Part model, mm, in its own coordinate system. A direction names the side the tool comes from. Coordinates: 2 decimals unless noted, no trailing zeros. Loops run counter-clockwise (first coordinate to the right, second up) from the corner with the lowest first, then second, coordinate; pieces in that order, holes last. Notation, with made-up numbers: (28, 10) - (45, 10) arc R26 cw to (45, 43) - close; hole circle Ø2 at (66.25, 46). An arc over 180 degrees is marked (long way). Use a Markdown table: item, result. Add a question column.
1) Band-saw the part on A-A (x = 5). Give the cut face in (y, z).
2) Probe probe 1 along Y at (x, z) = (0, -36.5); probe 2 along Z at (x, y) = (-2, 8); probe 3 along X at (y, z) = (-3.5, -16). List the from-to ranges inside material, lowest first. Write a range as [from, to].
3) Drop flat-ended pins along their axis: P1, Ø4.5, axis at x = 9.5, y = 0, coming from the +Z side; P2, Ø6.5, axis at x = 0, y = 10.5, coming from the +Z side; P3, Ø12, axis at x = 0.5, y = -0.5, coming from the -Z side; P4, Ø6, axis at x = -16, y = 10, coming from the +Z side. Give the stop position or say it passes through.
4) Pull direction Z, two halves, no side cores. Call faces 1 (the face through (-32, -7, -1)), 2 (the face through (10, 1, -13)), 3 (the face through (6.1, 10, -22)): +Z half, -Z half, draft (parallel to the pull), parting line (faces both ways), or undercut.
5) Band-saw the part on C-C (y = 4.25). Give the cut face in (x, z), plus the area to 3 significant figures.
6) Band-saw the part on D-D (z = -4). Give the cut face in (x, y).
7) Tool access for faces 4 (the face through (-13, -6.5, -3)), 5 (the face through (-13, 0, -13.3)), 6 (the face through (7, 0, -17.5)): list every direction of +Z, -Z, +X, -X, +Y, -Y with a clear straight run to the whole face (end or side of a thin tool).
8) Band-saw the part on B-B (z = -31). Give the cut face in (x, y), plus the area to 3 significant figures.
Autodesk Inventor part; units mm, degrees
ref_plane "作業平面2" through (0, 0, -13.3) normal (0, 0, 1) x (1, 0, 0)
ref_plane "作業平面3" through (0, 0, -9) normal (0, 0, 1) x (1, 0, 0)
ref_plane "作業平面4" through (-12.5, -8.5, -11.1) normal (-1, 0, 0) x (0, 0, 1)
sketch "スケッチ1" plane through (0, 0, 0) normal (0, 0, 1) x (1, 0, 0)
  circle A0 centre (0, 0) radius 1.5
  circle A1 centre (0, 0) radius 4
  line L0 (6.1, 4) -> (6.1, -4)
  line L1 (-27.76, 0) -> (17.46, 0) construction
  line L2 (6.1, 4) -> (0, 4)
  line L3 (6.1, -4) -> (0, -4)
  line L4 (6.1, -4) -> (8.1, -4)
  line L5 (8.1, -4) -> (8.1, 4)
  line L6 (8.1, 4) -> (6.1, 4)
  line L7 (0, -13.6) -> (0, 18.6) construction
  circle A2 centre (0, 10) radius 1.5
  circle A3 centre (0, 10) radius 4
  line L8 (6.1, 14) -> (6.1, 6)
  line L9 (6.1, 14) -> (0, 14)
  line L10 (6.1, 6) -> (0, 6)
  line L11 (6.1, 6) -> (8.1, 6)
  line L12 (8.1, 6) -> (8.1, 14)
  line L13 (8.1, 14) -> (6.1, 14)
  line L14 (-16.4, 6.05) -> (6.1, 6.05) construction
  line L15 (6.1, 6.05) -> (6.1, -6.05)
  line L16 (6.1, -6.05) -> (-16.4, -6.05) construction
  line L17 (-16.4, -6.05) -> (-16.4, 6.05)
  line L18 (-16.4, 6.05) -> (6.1, -6.05) construction
  line L19 (6.1, 6.05) -> (-16.4, -6.05) construction
  line L20 (-21.3, 6.05) -> (11, 6.05) construction
  line L21 (11, 6.05) -> (11, -6.05) construction
  line L22 (11, -6.05) -> (-21.3, -6.05)
  line L23 (-21.3, -6.05) -> (-21.3, 6.05) construction
  line L24 (-21.3, 6.05) -> (11, -6.05) construction
  line L25 (11, 6.05) -> (-21.3, -6.05) construction
  line L26 (-21.3, 0) -> (11, 0) construction
  circle A4 centre (-19, 0) radius 1.1
  line L27 (-5.15, 6.05) -> (-5.15, -6.05) construction
  circle A5 centre (0, 0) radius 2.425
  circle A6 centre (0, 0) radius 6.05
  circle A7 centre (0, 0) radius 9
  line L28 (8.1, -7) -> (-21.3, -7)
  line L29 (-21.3, -7) -> (-21.3, 6.05)
  line L30 (-21.3, 6.05) -> (8.1, 6.05)
  line L31 (8.1, 6.05) -> (8.1, -7)
  line L32 (-21.3, -5) -> (-20.943492, -5)
  line L33 (-20.943492, -5) -> (8.1, -5)
  circle A8 centre (8.7, 0) radius 1.1
  line L34 (8.1, 6.05) -> (11, 6.05)
  line L35 (11, 6.05) -> (11, -6.05)
  point P0 (6.1, 0)
  point P1 (6.1, 10)
  point P2 (-5.15, 0)
  point P3 (-5.15, 0)
  point P4 (-0.630476, 6.05)
  point P5 (8.1, 6.05)
  point P6 (8.1, -6.05)
  point P7 (0, 6.05)
  point P8 (-6.663145, 6.05)
  point P9 (-6.663145, -6.05)
  point P10 (0, -6.05)
  point P11 (6.1, 6.617401)
  point P12 (6.663145, 6.05)
  point P13 (0.630476, 6.05)
  point P14 (0.489992, 6.030125)
  point P15 (0.776209, 6)
  point P16 (8.062258, 4)
  point P17 (8.1, 3.923009)
  point P18 (8.062258, -4)
  point P19 (8.1, -3.923009)
  point P20 (6.708204, 6)
  dimension "d0" = 3
  dimension "d1" = 8
  dimension "d3" = 8
  dimension "d4" = 2
  dimension "d11" = 10
  dimension "d21" = 12.1
  dimension "d22" = 22.5
  dimension "d23" = 32.3
  dimension "d24" = 2.2
  dimension "d26" = 27.7
  dimension "d28" = 18
  dimension "d29" = 12.1
  dimension "d30" = 4.85
  dimension "d31" = 6.1
  dimension "d32" = 7
  dimension "d55" = 2
extrude "押し出し1" add sketch "スケッチ1" along normal blind 2 contours A1 | A1 L2 A6 L3 | L2 L0 L3 A6 | L6 A7 L5 A8 L4 L0 | L6 L5 A7 | A7 L5 L4 | L5 A8 | A5
extrude "押し出し2" add sketch "スケッチ1" against normal blind 7 contours L6 A7 L5 A8 L4 L0 | L6 L5 A7 | A7 L5 L4 | L5 A8
extrude "押し出し3" add sketch "スケッチ1" against normal blind 2 from surface at -7 contours A6 A3 L30 L8 L10 | L10 A3 A6 | L8 L30 A7 L11 | A3 A6 | A6 L30 A3 | A7 L30 L12 L11 | L30 A3 A7 L8 | L8 A7 L30 | A3 L30 A6 | L30 A3 A7 A2 | A7 L8 L13 L12 L30 | A7 A3 L9 L8 | A7 A2 A3
pattern_linear "矩形状パターン1" count 2 spacing 28 along (0, 0, -1) of "押し出し3"
ref_plane "作業平面1" through (0, 0, -17.5) normal (0, 0, 1) x (1, 0, 0)
extrude "押し出し4" add sketch "スケッチ1" against normal up to surface (10.5 mm away) from surface at -7 contours A0 | A1 | A1 L2 A6 L3 | A1 L3 A6 L33 A3 L10 L2 | A6 L10 L15 L2 | L2 L0 L3 A6 | L3 L15 L33 A6 | L6 A7 L5 A8 L4 L0 | L15 L11 A7 L6 | A6 A3 L30 L8 L10 | L10 A3 A6 | L4 A7 L33 L15 | L33 L15 L22 A6 | A6 L33 | A7 L11 L31 L6 | L6 L5 A7 | L8 L30 A7 L11 | A3 A6 | A6 L30 A3 | A7 L5 L4 | L4 L31 L33 A7 | L33 A7 L22 L15 | L22 A7 L28 | L22 A7 L33 A6 | L33 A7 L30 A3 A6 | A7 L30 L12 L11 | A3 L30 A6 | L33 L31 L22 A7 | A7 L28 L29 L22 | L22 L17 L33 A7 | L33 L17 L30 A7 | L5 A8 | L22 L31 L28 A7 | L22 L29 L32 L33 L17 | L33 L32 L29 L30 L17 | A4 | A5
ref_plane "作業平面2" through (0, 0, -13.3) normal (0, 0, 1) x (1, 0, 0)
extrude "押し出し6" cut sketch "スケッチ1" against normal blind 23.4 from surface at -13.3 contours A0 | A1 | A1 L2 A6 L3 | A1 L3 A6 L33 A3 L10 L2 | A6 L10 L15 L2 | L2 L0 L3 A6 | L3 L15 L33 A6 | A6 A3 L30 L8 L10 | L10 A3 A6 | L33 L15 L22 A6 | A6 L33 | A3 A6 | A6 L30 A3 | L22 A7 L33 A6 | L33 A7 L30 A3 A6 | A3 L30 A6 | L22 L17 L33 A7 | L33 L17 L30 A7 | A5
ref_plane "作業平面3" through (0, 0, -9) normal (0, 0, 1) x (1, 0, 0)
extrude "押し出し7" cut sketch "スケッチ1" against normal up to surface (4.3 mm away) from surface at -9 contours A0 | A1 | A1 L2 A6 L3 | A1 L3 A6 L33 A3 L10 L2 | L10 A3 A6 | A6 L33 | A3 A6 | L22 A7 L33 A6 | L33 A7 L30 A3 A6 | A3 L30 A6 | A5 picked at (-0.459231, 6.046871)
extrude "押し出し8" cut sketch "スケッチ1" against normal up to surface (9 mm away) contours A0 | A5
extrude "押し出し9" cut sketch "スケッチ1" against normal through all contours A4
extrude "押し出し10" add sketch "スケッチ1" against normal up to surface (28 mm away) from surface at -9 contours L22 A7 L28 | L8 A7 L30 | A7 L28 L29 L22 | A7 L8 L13 L12 L30 | L22 L31 L28 A7
extrude "押し出し11" cut sketch "スケッチ1" against normal up to surface (19.5 mm away) from surface at -17.5 contours A6 A3 L30 L8 L10 | L10 A3 A6 | L8 L30 A7 L11 | A3 A6 | A6 L30 A3 | A7 L30 L12 L11 | A3 L30 A6
sketch "スケッチ3" plane through (0, 4, 2) normal (0, 1, 0) x (1, 0, 0)
  line L0 (8.1, 0) -> (0, 0)
  line L1 (8.1, 9) -> (8.1, 0)
  line L2 (6.1, 9) -> (8.1, 9)
  line L3 (6.1, 2) -> (6.1, 9)
  line L4 (6.1, 2) -> (0, 2)
  line L5 (0, 2) -> (0, 0)
  line L6 (0, 2) -> (0, 2)
  line L7 (0, 2) -> (0, 0)
  line L8 (0, 0) -> (0, 0)
  line L9 (0, 2) -> (0, 0)
  line L10 (-4, 2) -> (-4, 0)
  line L11 (-4, 2) -> (0, 2)
  line L12 (-4, 0) -> (0, 0)
extrude "押し出し12" cut sketch "スケッチ3" against normal through all
extrude "押し出し13" add sketch "スケッチ1" along normal blind 10 and the other way blind 7 contours L33 L15 L22 A6 | A6 L33 | L33 A7 L22 L15 | L22 A7 L28 | L22 A7 L33 A6 | L33 L31 L22 A7 | A7 L28 L29 L22 | L22 L17 L33 A7 | L22 L31 L28 A7 | L22 L29 L32 L33 L17
sketch "スケッチ4" plane through (-21.3, 6.05, -17.5) normal (-1, 0, 0) x (0, 0, 1)
  line L0 (27.5, -13.05) -> (-19.5, -13.05)
  line L1 (27.5, -11.05) -> (27.5, -13.05)
  line L2 (10.5, -11.05) -> (27.5, -11.05)
  line L3 (10.5, 0) -> (10.5, -11.05)
  line L4 (10.5, 0) -> (0, 0)
  line L5 (0, -12.1) -> (0, 0)
  line L6 (0, -12.1) -> (-19.5, -12.1)
  line L7 (-19.5, -12.1) -> (-19.5, -13.05)
  line L8 (10.5, -11.05) -> (10.5, -13.05)
  point P0 (17.5, -6.05)
extrude "押し出し14" add sketch "スケッチ4" along normal blind 10.7 contours L0 L8 L2 L1
sketch "スケッチ5" plane through (-21.3, -5, -47) normal (0, -1, 0) x (1, 0, 0)
  line L0 (29.4, 10) -> (29.4, 57)
  line L1 (29.4, 57) -> (-10.7, 57)
  line L2 (-10.7, 40) -> (-10.7, 57)
  line L3 (0, 40) -> (-10.7, 40)
  line L4 (0, 40) -> (0, 10)
  line L5 (0, 10) -> (29.4, 10)
  line L6 (-10.7, 43.5) -> (29.4, 43.5) construction
  line L7 (1.2, 51.1) -> (16.4, 51.1)
  line L8 (16.4, 51.1) -> (16.4, 35.9)
  line L9 (16.4, 35.9) -> (1.2, 35.9)
  line L10 (1.2, 35.9) -> (1.2, 51.1)
  line L11 (1.2, 51.1) -> (16.4, 35.9) construction
  line L12 (16.4, 51.1) -> (1.2, 35.9) construction
  line L13 (-10.7, 57) -> (-10.7, 40)
  line L14 (-10.7, 40) -> (-10.7, 33.9)
  line L15 (-10.7, 33.9) -> (0, 33.9)
  line L16 (29.4, 57) -> (-10.7, 57)
  point P0 (21.3, 47)
  point P1 (8.8, 43.5)
  dimension "d63" = 15.2
  dimension "d64" = 15.2
  dimension "d68" = 13.5
  dimension "d69" = 2
  dimension "d105" = 19.5
extrude "押し出し17" add sketch "スケッチ5" along normal blind 1.5 from surface at 2 contours L5 L4 L3 L2 L1 L0 | L7 L8 L9 L10
extrude "押し出し15" cut sketch "スケッチ5" against normal blind 2 from surface at 3.5 contours L7 L8 L9 L10
ref_plane "作業平面4" through (-12.5, -8.5, -11.1) normal (-1, 0, 0) x (0, 0, 1)
ref_plane "作業平面5" through (-20.1, -6.5, -3.5) normal (0, 0, 1) x (1, 0, 0)
extrude "押し出し16" add sketch "スケッチ5" along normal up to surface (3.5 mm away) contours L15 L14 L3 L4
extrude "押し出し18" add sketch "スケッチ1" against normal up to surface (10.5 mm away) from surface at -7 contours L6 A7 L5 A8 L4 L0 | L15 L11 A7 L6 | L4 A7 L33 L15 | A7 L11 L31 L6 | L4 L31 L33 A7 | L33 A7 L22 L15 | L31 L12 L34 L35 L22 L5 A7 A8 | A7 A8 L5 | A7 L30 L12 L11 | L33 L31 L22 A7 | L5 A8 A7 | A8 A7 L5 | L5 A8 | A8 A7
extrude "押し出し19" cut sketch "スケッチ1" against normal through all contours A8 A7 L5 | L5 A8 | A8 A7 picked at (8.4, 0)
sketch "スケッチ6" plane through (8.1, -5, 10) normal (1, 0, 0) x (0, 0, -1)
  line L0 (27.5, -1.05) -> (17, -1.05)
  line L1 (17, -1.05) -> (17, 0)
  line L2 (17, 0) -> (0, 0)
  line L3 (0, 0) -> (0, -3.5)
  line L4 (0, -3.5) -> (47, -3.5)
  line L5 (47, -1.05) -> (47, -3.5)
  line L6 (27.5, -1.05) -> (47, -1.05)
  point P0 (10, 5)
extrude "押し出し20" add sketch "スケッチ6" along normal up to surface (2.9 mm away)
sketch "スケッチ7" plane through (6.1, -6.05, -17.5) normal (0, 0, -1) x (-1, 0, 0)
  circle A0 centre (-2.6, 6.05) radius 1.1
  line L0 (-4.9, 0) -> (0, 0)
  line L1 (0, 0) -> (0, 12.1)
  line L2 (0, 12.1) -> (-2, 12.1)
  line L3 (-2, 12.1) -> (-4.9, 12.1)
  line L4 (-4.9, 12.1) -> (-4.9, 0)
  line L5 (0, 12.1) -> (0, 0)
  line L6 (0, 0) -> (6.1, 0)
  arc A1 (6.1, 12.1) -> (6.1, 0) centre (6.1, 6.05) ccw
  line L7 (0, 12.1) -> (6.1, 12.1)
  arc A2 (12.763145, 0) -> (12.763145, 12.1) centre (6.1, 6.05) ccw
  line L8 (12.763145, 0) -> (22.5, 0)
  line L9 (22.5, 0) -> (22.5, 12.1)
  line L10 (12.763145, 12.1) -> (22.5, 12.1)
  line L11 (22.5, 12.1) -> (22.5, 0)
  line L12 (22.5, 0) -> (27.4, 0)
  line L13 (27.4, 0) -> (27.4, 12.1)
  line L14 (27.4, 12.1) -> (22.5, 12.1)
  circle A3 centre (25.1, 6.05) radius 1.1
  line L15 (6.730476, 12.1) -> (12.763145, 12.1)
  line L16 (6.1, 0) -> (12.763145, 0)
  circle A4 centre (6.1, 6.05) radius 2.425
  line L17 (0, 12.1) -> (6.1, 12.1)
  line L18 (6.1, 12.1) -> (6.730476, 12.1)
  line L19 (-0.1, 12.1) -> (-0.1, 0)
  line L20 (-4.9, 0) -> (0, 0)
  line L21 (22.6, 12.1) -> (22.6, 0)
  line L22 (22.5, 0) -> (27.4, 0)
  arc A5 (6.1, 12.2) -> (6.1, -0.1) centre (6.1, 6.05) ccw
  arc A6 (12.83718, -0.067222) -> (12.83718, 12.167222) centre (6.1, 6.05) ccw
  circle A7 centre (6.1, 6.05) radius 3.7
  line L23 (15.2, 12.1) -> (15.2, 0)
  line L24 (27.4, 1.05) -> (-4.9, 1.05)
  line L25 (23.1, 1.05) -> (23.1, 12.1)
  line L26 (-0.6, 1.05) -> (-0.6, 12.1)
  line L27 (22.5, 12.1) -> (22.5, 0)
  line L28 (22.5, 0) -> (27.4, 0)
  line L29 (27.4, 0) -> (27.4, 12.1)
  line L30 (27.4, 12.1) -> (22.5, 12.1)
  point P0 (22.6, 0)
  point P1 (-0.1, 0)
  point P2 (12.89761, 0)
  point P3 (12.89761, 12.1)
  point P4 (4.995464, 12.1)
  point P5 (4.995464, 0)
  point P6 (15.2, 6.05)
  dimension "d80" = 0.1
  dimension "d81" = 0.1
  dimension "d84" = 0.1
  dimension "d85" = 0.1
  dimension "d99" = 2
  dimension "d101" = 2
  dimension "d104" = 7.4
extrude "押し出し21" cut sketch "スケッチ7" against normal up to surface (4.2 mm away) contours L19 L24 L1 L0 | L19 L2 L1 A5 L24 | A5 L1 | L9 L24 L21 L12 | L9 L14 L21 L24
sketch "スケッチ7 outline for 押し出し22" plane through (6.1, -6.05, -17.5) normal (0, 0, -1) x (-1, 0, 0)
  arc A0 (12.763145, 12.1) -> (12.763145, 0) centre (6.1, 6.05) cw
  line L0 (12.763145, 0) -> (15.2, 0)
  line L1 (15.2, 0) -> (15.2, 12.1)
  line L2 (15.2, 12.1) -> (12.763145, 12.1)
  arc A1 (6.1, 0) -> (6.1, 12.1) centre (6.1, 6.05) cw
  line L3 (6.1, 12.1) -> (-0.1, 12.1)
  line L4 (-0.1, 12.1) -> (-0.1, 0)
  line L5 (-0.1, 0) -> (6.1, 0)
extrude "押し出し22" cut sketch "スケッチ7 outline for 押し出し22" against normal up to surface (8.5 mm away)
extrude "押し出し23" cut sketch "スケッチ7" against normal through all contours A7
extrude "押し出し26" cut sketch "スケッチ7" along normal blind 6 from surface at -10.5 contours L4 L3 L2 L26 L24 | L25 L14 L13 L24
properties part number "housing_shaft_link_base"
Answer block:
| question | item | result |
|---|---|---|
| 1 | outline | (-8.5, -37) - (-6.05, -37) - (-6.05, -9) - (14, -9) - (14, -7) - (-5, -7) - (-5, 10) - (-8.5, 10) - close; (6.05, -37) - (14, -37) - (14, -35) - (6.05, -35) - close |
| 2 | probe 1 | [-8.5, -6.05], [6.05, 8.5], [11.5, 14] |
| 2 | probe 2 | [-37, -35], [-9, -7] |
| 2 | probe 3 | [-21.3, -16.5], [6.2, 11] |
| 3 | P1 | z = -13 |
| 3 | P2 | z = -7 |
| 3 | P3 | z = -37 |
| 3 | P4 | through |
| 4 | face 1 | draft |
| 4 | face 2 | +Z half |
| 4 | face 3 | undercut |
| 5 | outline | (-21.3, -17.5) - (-16.5, -17.5) - (-16.5, -13.3) - (-9.1, -13.3) - (-9.1, -9) - (6.2, -9) - (6.2, -17.5) - (11, -17.5) - (11, -13) - (6.7, -13) - (6.7, -7) - (-17, -7) - (-17, -13) - (-21.3, -13) - close |
| 5 | area | 126 mm2 |
| 6 | outline | (-32, -8.5) - (-20.1, -8.5) - (-20.1, -6.5) - (-4.9, -6.5) - (-4.9, -8.5) - (11, -8.5) - (11, -5) - (-32, -5) - close |
| 7 | face 4 | -Y |
| 7 | face 5 | -Z, +Y |
| 7 | face 6 | -Z, +X, -X |
| 8 | outline | (-21.3, -8.5) - (11, -8.5) - (11, -6.05) - (-21.3, -6.05) - close; (6.1, 6.05) - (8.1, 6.05) - (8.1, 14) - (6.1, 14) - close |
| 8 | area | 95.0 mm2 |
